from build123d import *

# Parameters (mm, degrees)
SKETCH1_R               = 55
BOSS_EXTRUDE1_DEPTH     = 15.5
SKETCH2_R               = 44.25
BOSS_EXTRUDE2_DEPTH     = 15
CUT_EXTRUDE3_DEPTH      = 84.547890458
CUT_EXTRUDE3_DEPTH_BACK = 84.547890458
SKETCH3_R               = 37.5


with BuildPart() as part:
    # Sketch1 → Boss-Extrude1 (new body)
    with BuildSketch(Plane.XY):
        Circle(SKETCH1_R)
    extrude(amount=BOSS_EXTRUDE1_DEPTH)

    # Sketch2 → Boss-Extrude2 (add)
    with BuildSketch(Plane.XY.offset(15.5)):
        Circle(SKETCH2_R)
    extrude(amount=BOSS_EXTRUDE2_DEPTH)

    # Sketch3 → Cut-Extrude3 (cut, two sides: drawn at the far end of the back side and taken through both)
    with BuildSketch(Plane(origin=(0, 0, 0), x_dir=(-1, 0, 0), z_dir=(0, 0, -1)).offset(-CUT_EXTRUDE3_DEPTH_BACK)):
        Circle(SKETCH3_R)
    extrude(amount=CUT_EXTRUDE3_DEPTH + CUT_EXTRUDE3_DEPTH_BACK, mode=Mode.SUBTRACT)


solid = part.part
The listing builds one solid part. Answer for the finished solid, in the listing's coordinates (mm). A direction names the side the tool comes from. Round coordinates to 2 decimals unless told otherwise and drop trailing zeros. Write each loop counter-clockwise with the first axis right and the second up, starting at its lowest first coordinate (ties: lowest second). Pieces come first, ordered by that corner, then holes. Notation, with made-up numbers: M 39.5,-30 L 80.5,-30 A11 cw 80.5,-16 Z; hole C -25,-21.5 d11. An arc over 180 degrees is marked long. Write each question's results on one line, items separated by ' | '. Start each with the question number.
Item 1: Find section B-B on x = -31. Write down the section's boundary in (y, z), and give its area (3 significant figures).
Item 2: Which of the six approach directions +Z, -Z, +X, -X, +Y, -Y give full straight-line access (tool end or side, diameter ignored) to faces 1 (the flat face through (11.5, -35.9, 0)), 2 (the flat face through (-37, 25, 15.5))?
Item 3: Straight lines are drawn through the part: probe 1 along Y at (x, z) = (0, 17); probe 2 along Y at (x, z) = (0, 13); probe 3 along Z at (x, y) = (44, -14). For each, find the intervals that lie inside material, in ascending order.
Item 4: Find section A-A on y = 0. Write down the section's boundary in (x, z).
Item 5: Given pin 1 Ø1 at (y, z) = (-38, 19) entering from +X; pin 2 Ø1.5 at (y, z) = (10.5, 18.5) entering from +X; pin 3 Ø8 at (x, z) = (3, 13) entering from +Y, each flat-ended and moving along its own axis, determine where each tip first touches the part or whether it passes through.
Item 6: The mould has two halves that part along Y. Classify faces 3 (the cylindrical face through (-11.923, -53.692, 7.642)), 4 (the cylindrical face through (4.88, 37.18, 15.46)), 5 (the flat face through (-36.3, 10, 30.5)): +Y half, -Y half, draft (parallel to the pull), parting line (faces both ways), or undercut.
Item 7: Find section D-D on z = 6.5. Write down the section's boundary in (x, y).
Item 8: Find section C-C on z = 23.5. Write down the section's boundary in (x, y).
Answer block:
1) outline: M -45.43,0 L -21.1,0 L -21.1,30.5 L -31.58,30.5 L -31.58,15.5 L -45.43,15.5 Z; M 21.1,0 L 45.43,0 L 45.43,15.5 L 31.58,15.5 L 31.58,30.5 L 21.1,30.5 Z | area: 1,070 mm²
2) face 1: -Z, +X, -X, +Y, -Y | face 2: +Z
3) probe 1: y = -44.25 to -37.5, 37.5 to 44.25 | probe 2: y = -55 to -37.5, 37.5 to 55 | probe 3: z = 0 to 15.5
4) outline: M -55,0 L -37.5,0 L -37.5,30.5 L -44.25,30.5 L -44.25,15.5 L -55,15.5 Z; M 37.5,0 L 55,0 L 55,15.5 L 44.25,15.5 L 44.25,30.5 L 37.5,30.5 Z
5) pin 1: stops at x = 23.49 | pin 2: stops at x = 43.16 | pin 3: stops at y = 55
6) face 3: parting line | face 4: undercut | face 5: draft
7) outline: C 0,0 d110; hole C 0,0 d75
8) outline: C 0,0 d88.5; hole C 0,0 d75
